Source: CAD feature listing. Evaluate the final solid. Frame: model axes, mm. Face numbers are marked on the shaded views. A direction names the side the tool comes from. Coordinates: 2 decimals unless noted, no trailing zeros. Write each loop counter-clockwise with the first axis right and the second up, starting at its lowest first coordinate (ties: lowest second). Pieces come first, ordered by that corner, then holes. Notation, with made-up numbers: M 30.5,66 L 65.5,66 A34 ccw 65.5,103 Z; hole C -4.75,13 d6. An arc over 180 degrees is marked long. Write item = value, one per line. Start each with the question number.
1. Pull-direction query (Y, two-part tool) for the marked faces 3, 4 and 5; classes: pulls with the +Y half, pulls with the -Y half, needs draft (parallel to the pull), parting line crosses it, or undercut.
2. Section query B-B (z = 32). Output: boundary loops of the cut face in (x, y).
3. Pin query (flat end, axial travel): pin 1 Ø6 at (x, z) = (-34, 56) entering from -Y. Return the tip coordinate at first contact, or that it passes through.
4. Section query C-C (y = -42.5). Output: boundary loops of the cut face in (x, z), then the cut area to 3 significant figures.
5. Access query for the marked faces 1 and 2. Directions: +Z, -Z, +X, -X, +Y, -Y. A direction counts if a zero-diameter tool reaches every point of the face in a straight line with its end or side. Return the directions, or none.
6. Line query: line 1 along X through (y, z) = (-19.5, 97); line 2 along X through (y, z) = (-48, 44). Output: solid intervals per line, ascending.
7. Section query A-A (x = -34). Output: boundary loops of the cut face in (y, z), then the cut area to 3 significant figures.
```python
from build123d import *

# Parameters (mm, degrees)
SKETCH1_W                      = 100
SKETCH1_H                      = 100
SKETCH1_W_2                    = 94
SKETCH1_H_2                    = 94
EXTRUDE_THIN1_DEPTH            = 130
FILLET1_R                      = 0.5
FILLET2_R                      = 3
F_8_0_8_DIAMETER_HOLE2_D       = 8
F_8_0_8_DIAMETER_HOLE3_D       = 8
F_10_0_10_DIAMETER_HOLE1_D     = 10
F_10_0_10_DIAMETER_HOLE2_D     = 10
M8X1_25_TAPPED_HOLE1_D         = 6.8
M8X1_25_TAPPED_HOLE1_DEPTH     = 3
M8X1_25_TAPPED_HOLE2_D         = 6.8
M8X1_25_TAPPED_HOLE2_DEPTH     = 3
F_21_0_21_DIAMETER_HOLE1_D     = 21
F_21_0_21_DIAMETER_HOLE1_DEPTH = 3
F_6_0_6_DIAMETER_HOLE1_D       = 6
F_6_0_6_DIAMETER_HOLE1_DEPTH   = 3
F_8_0_8_DIAMETER_HOLE4_D       = 8
F_8_0_8_DIAMETER_HOLE4_DEPTH   = 3
CUT_EXTRUDE1_REACH             = 173.464
SKETCH31_R                     = 2
SKETCH31_R_2                   = 3.5


with BuildPart() as part:
    # Sketch1 → Extrude-Thin1 (new body)
    with BuildSketch(Plane.XY):
        Rectangle(SKETCH1_W, SKETCH1_H)
        Rectangle(SKETCH1_W_2, SKETCH1_H_2, mode=Mode.SUBTRACT)
    extrude(amount=EXTRUDE_THIN1_DEPTH)

    # Fillet1
    fillet1_edges = [part.edges().sort_by_distance(p)[0] for p in [
        (47, -47, 65),
        (47, 47, 65),
        (-47, 47, 65),
        (-47, -47, 65),
    ]]
    fillet(fillet1_edges, radius=FILLET1_R)

    # Fillet2
    fillet2_edges = [part.edges().sort_by_distance(p)[0] for p in [
        (50, -50, 65),
        (-50, -50, 65),
        (-50, 50, 65),
        (50, 50, 65),
    ]]
    fillet(fillet2_edges, radius=FILLET2_R)

    # Ø8.0 (8) Diameter Hole2 (through all)
    with Locations(Plane(origin=(0, 50, 0), x_dir=(1, 0, 0), z_dir=(0, 1, 0))):
        with Locations((28, -32), (28, -90)):
            Hole(F_8_0_8_DIAMETER_HOLE2_D / 2)

    # Ø8.0 (8) Diameter Hole3 (through all)
    with Locations(Plane(origin=(50, 0, 0), x_dir=(0, 0, -1), z_dir=(1, 0, 0))):
        with Locations((-14, 31), (-110, 31)):
            Hole(F_8_0_8_DIAMETER_HOLE3_D / 2)

    # Ø10.0 (10) Diameter Hole1 (through all)
    with Locations(Plane(origin=(0, 50, 0), x_dir=(1, 0, 0), z_dir=(0, 1, 0))):
        with Locations((-34, -56)):
            Hole(F_10_0_10_DIAMETER_HOLE1_D / 2)

    # Ø10.0 (10) Diameter Hole2 (through all)
    with Locations(Plane(origin=(50, 0, 0), x_dir=(0, 0, -1), z_dir=(1, 0, 0))):
        with Locations((-44, -31)):
            Hole(F_10_0_10_DIAMETER_HOLE2_D / 2)

    # M8x1.25 Tapped Hole1
    with Locations(Plane.ZY.offset(50)):
        with Locations((56, -15), (56, 35)):
            Hole(M8X1_25_TAPPED_HOLE1_D / 2, depth=M8X1_25_TAPPED_HOLE1_DEPTH)

    # M8x1.25 Tapped Hole2
    with Locations(Plane(origin=(0, -50, 0), x_dir=(-1, 0, 0), z_dir=(0, -1, 0))):
        with Locations((20, -44), (-35, -44)):
            Hole(M8X1_25_TAPPED_HOLE2_D / 2, depth=M8X1_25_TAPPED_HOLE2_DEPTH)

    # Ø21.0 (21) Diameter Hole1
    with Locations(Plane(origin=(50, 0, 0), x_dir=(0, 0, -1), z_dir=(1, 0, 0))):
        with Locations((-70, 0)):
            Hole(F_21_0_21_DIAMETER_HOLE1_D / 2, depth=F_21_0_21_DIAMETER_HOLE1_DEPTH)

    # Ø6.0 (6) Diameter Hole1
    with Locations(Plane(origin=(50, 0, 0), x_dir=(0, 0, -1), z_dir=(1, 0, 0))):
        with Locations((-41.157258279, -16.652364697), (-53.347635303, 28.842741721), (-98.842741721, 16.652364697), (-86.652364697, -28.842741721)):
            Hole(F_6_0_6_DIAMETER_HOLE1_D / 2, depth=F_6_0_6_DIAMETER_HOLE1_DEPTH)

    # Ø8.0 (8) Diameter Hole4
    with Locations(Plane(origin=(0, 50, 0), x_dir=(1, 0, 0), z_dir=(0, 1, 0))):
        with Locations((-3, -24)):
            Hole(F_8_0_8_DIAMETER_HOLE4_D / 2, depth=F_8_0_8_DIAMETER_HOLE4_DEPTH)

    # Sketch31 → Cut-Extrude1 (cut, up to next)
    with BuildSketch(Plane(origin=(50, 0, 0), x_dir=(0, 0, -1), z_dir=(1, 0, 0)), mode=Mode.PRIVATE) as cut_extrude1_sk1:
        with Locations(Location((-5, 4, 0), (0, 0, 90))):
            Circle(SKETCH31_R)
    cut_extrude1_tool1 = extrude(cut_extrude1_sk1.sketch, amount=-CUT_EXTRUDE1_REACH, mode=Mode.PRIVATE) & part.part
    # Sketch31 → Cut-Extrude1 (cut, up to next)
    with BuildSketch(Plane(origin=(50, 0, 0), x_dir=(0, 0, -1), z_dir=(1, 0, 0)), mode=Mode.PRIVATE) as cut_extrude1_sk2:
        with Locations(Location((-5, 13, 0), (0, 0, 90))):
            Circle(SKETCH31_R)
    cut_extrude1_tool2 = extrude(cut_extrude1_sk2.sketch, amount=-CUT_EXTRUDE1_REACH, mode=Mode.PRIVATE) & part.part
    # Sketch31 → Cut-Extrude1 (cut, up to next)
    with BuildSketch(Plane(origin=(50, 0, 0), x_dir=(0, 0, -1), z_dir=(1, 0, 0)), mode=Mode.PRIVATE) as cut_extrude1_sk3:
        with Locations(Location((-125, 13, 0), (0, 0, 90))):
            Circle(SKETCH31_R)
    cut_extrude1_tool3 = extrude(cut_extrude1_sk3.sketch, amount=-CUT_EXTRUDE1_REACH, mode=Mode.PRIVATE) & part.part
    # Sketch31 → Cut-Extrude1 (cut, up to next)
    with BuildSketch(Plane(origin=(50, 0, 0), x_dir=(0, 0, -1), z_dir=(1, 0, 0)), mode=Mode.PRIVATE) as cut_extrude1_sk4:
        with Locations(Location((-125, 4, 0), (0, 0, 90))):
            Circle(SKETCH31_R)
    cut_extrude1_tool4 = extrude(cut_extrude1_sk4.sketch, amount=-CUT_EXTRUDE1_REACH, mode=Mode.PRIVATE) & part.part
    # Sketch31 → Cut-Extrude1 (cut, up to next)
    with BuildSketch(Plane(origin=(50, 0, 0), x_dir=(0, 0, -1), z_dir=(1, 0, 0)), mode=Mode.PRIVATE) as cut_extrude1_sk5:
        with Locations(Location((-23, 8.5, 0), (0, 0, 90))):
            Circle(SKETCH31_R_2)
    cut_extrude1_tool5 = extrude(cut_extrude1_sk5.sketch, amount=-CUT_EXTRUDE1_REACH, mode=Mode.PRIVATE) & part.part
    # Sketch31 → Cut-Extrude1 (cut, up to next)
    with BuildSketch(Plane(origin=(50, 0, 0), x_dir=(0, 0, -1), z_dir=(1, 0, 0)), mode=Mode.PRIVATE) as cut_extrude1_sk6:
        with Locations(Location((-107, 8.5, 0), (0, 0, 90))):
            Circle(SKETCH31_R_2)
    cut_extrude1_tool6 = extrude(cut_extrude1_sk6.sketch, amount=-CUT_EXTRUDE1_REACH, mode=Mode.PRIVATE) & part.part
    add(cut_extrude1_tool1.solids().sort_by_distance((50, 4, 5))[0], mode=Mode.SUBTRACT)
    add(cut_extrude1_tool2.solids().sort_by_distance((50, 13, 5))[0], mode=Mode.SUBTRACT)
    add(cut_extrude1_tool3.solids().sort_by_distance((50, 13, 125))[0], mode=Mode.SUBTRACT)
    add(cut_extrude1_tool4.solids().sort_by_distance((50, 4, 125))[0], mode=Mode.SUBTRACT)
    add(cut_extrude1_tool5.solids().sort_by_distance((50, 8.5, 23))[0], mode=Mode.SUBTRACT)
    add(cut_extrude1_tool6.solids().sort_by_distance((50, 8.5, 107))[0], mode=Mode.SUBTRACT)


solid = part.part
```
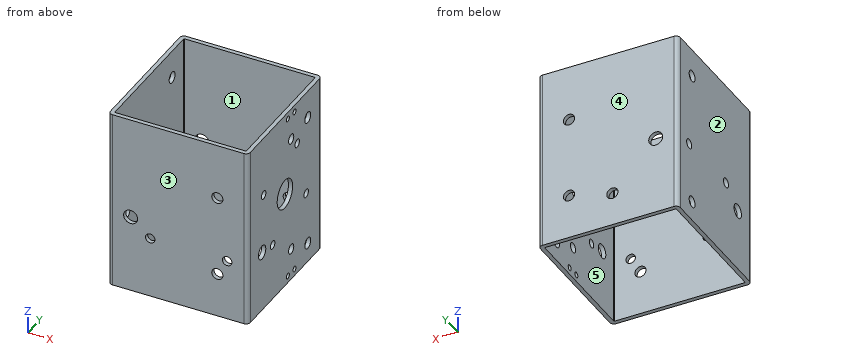
Results are:
q1.face_3 = pulls with the -Y half
q1.face_4 = pulls with the +Y half
q1.face_5 = undercut
q2.outline = M -50,-47 A3 ccw -47,-50 L 24,-50 L 24,-47 L -46.5,-47 A0.5 cw -47,-46.5 L -47,46.5 A0.5 cw -46.5,47 L 24,47 L 24,50 L -47,50 A3 ccw -50,47 Z; M 32,-50 L 47,-50 A3 ccw 50,-47 L 50,47 A3 ccw 47,50 L 32,50 L 32,47 L 46.5,47 A0.5 cw 47,46.5 L 47,-46.5 A0.5 cw 46.5,-47 L 32,-47 Z
q3.pin_1 = through
q4.outline = M -50,0 L -47,0 L -47,130 L -50,130 Z; M 47,0 L 50,0 L 50,130 L 47,130 Z
q4.area = 780 mm^2
q5.face_1 = +Z, -Z
q5.face_2 = +Z, -Z, -X, +Y, -Y
q6.line_1 = -50 to -47, 47 to 50
q6.line_2 = -49.83 to -23.4, -16.6 to 31.6, 38.4 to 49.83
q7.outline = M -50,0 L -47,0 L -47,51 L -50,51 Z; M -50,61 L -47,61 L -47,130 L -50,130 Z; M 47,0 L 50,0 L 50,51 L 47,51 Z; M 47,61 L 50,61 L 50,130 L 47,130 Z
q7.area = 720 mm^2
